```python
from build123d import *

# Parameters (mm, degrees)
F0_W     = 33.02
F0_H     = 17.78
F1_DEPTH = 1.6
F2_R     = 0.5
F3_DEPTH = 25


with BuildPart() as f1:
    # F0 (on Top) → F1 (new body)
    with BuildSketch(Plane.XY):
        Rectangle(F0_W, F0_H)
    extrude(amount=F1_DEPTH)

    # F2 (on Top) → F3 (cut)
    with BuildSketch(Plane.XY):
        with Locations((-12.974238, 7.62)):
            Circle(F2_R)
        with Locations((-10.434238, 7.62)):
            Circle(F2_R)
        with Locations((-7.894238, 7.62)):
            Circle(F2_R)
        with Locations((-5.354238, 7.62)):
            Circle(F2_R)
        with Locations((-2.814238, 7.62)):
            Circle(F2_R)
        with Locations((-0.274238, 7.62)):
            Circle(F2_R)
        with Locations((2.265762, 7.62)):
            Circle(F2_R)
        with Locations((4.805762, 7.62)):
            Circle(F2_R)
        with Locations((7.345762, 7.62)):
            Circle(F2_R)
        with Locations((9.885762, 7.62)):
            Circle(F2_R)
        with Locations((12.425762, 7.62)):
            Circle(F2_R)
        with Locations((14.965762, 7.62)):
            Circle(F2_R)
        with Locations((2.265762, -7.62)):
            Circle(F2_R)
        with Locations((4.805762, -7.62)):
            Circle(F2_R)
        with Locations((7.345762, -7.62)):
            Circle(F2_R)
        with Locations((9.885762, -7.62)):
            Circle(F2_R)
        with Locations((12.425762, -7.62)):
            Circle(F2_R)
        with Locations((-0.274238, -7.62)):
            Circle(F2_R)
        with Locations((14.965762, -7.62)):
            Circle(F2_R)
        with Locations((-2.814238, -7.62)):
            Circle(F2_R)
        with Locations((-7.894238, -7.62)):
            Circle(F2_R)
        with Locations((-12.974238, -7.62)):
            Circle(F2_R)
        with Locations((-5.354238, -7.62)):
            Circle(F2_R)
        with Locations((-10.434238, -7.62)):
            Circle(F2_R)
    extrude(amount=F3_DEPTH, mode=Mode.SUBTRACT)


solid = f1.part
```
Input: part model. Units: mm. Frame: model coordinates. Coordinates: 2 decimals unless noted, no trailing zeros.
1) Section A-A on z = 1.25. State how many separate pieces and enclosed holes the cut face has, and give its area (3 significant figures).
2) Mould query, pull axis X, two halves, no side actions, for faces 1 (the cylindrical face through (7.24, 7.13, 0.79)), 2 (the flat face through (0, -8.89, 1)). Classes: pulls with the +X half, pulls with the -X half, needs draft (parallel to the pull), parting line crosses it, or undercut.
3) Material intervals for line 1 along Y through (x, z) = (15, 1.1); line 2 along Y through (x, z) = (5, 1.4), sorted ascending.
Check result:
1. separate pieces: 1
1. enclosed holes: 24
1. area: 568 mm2
2. face 1: undercut
2. face 2: needs draft
3. line 1: y = -8.89 to -8.12, -7.12 to 7.12, 8.12 to 8.89
3. line 2: y = -8.89 to -8.08, -7.16 to 7.16, 8.08 to 8.89
